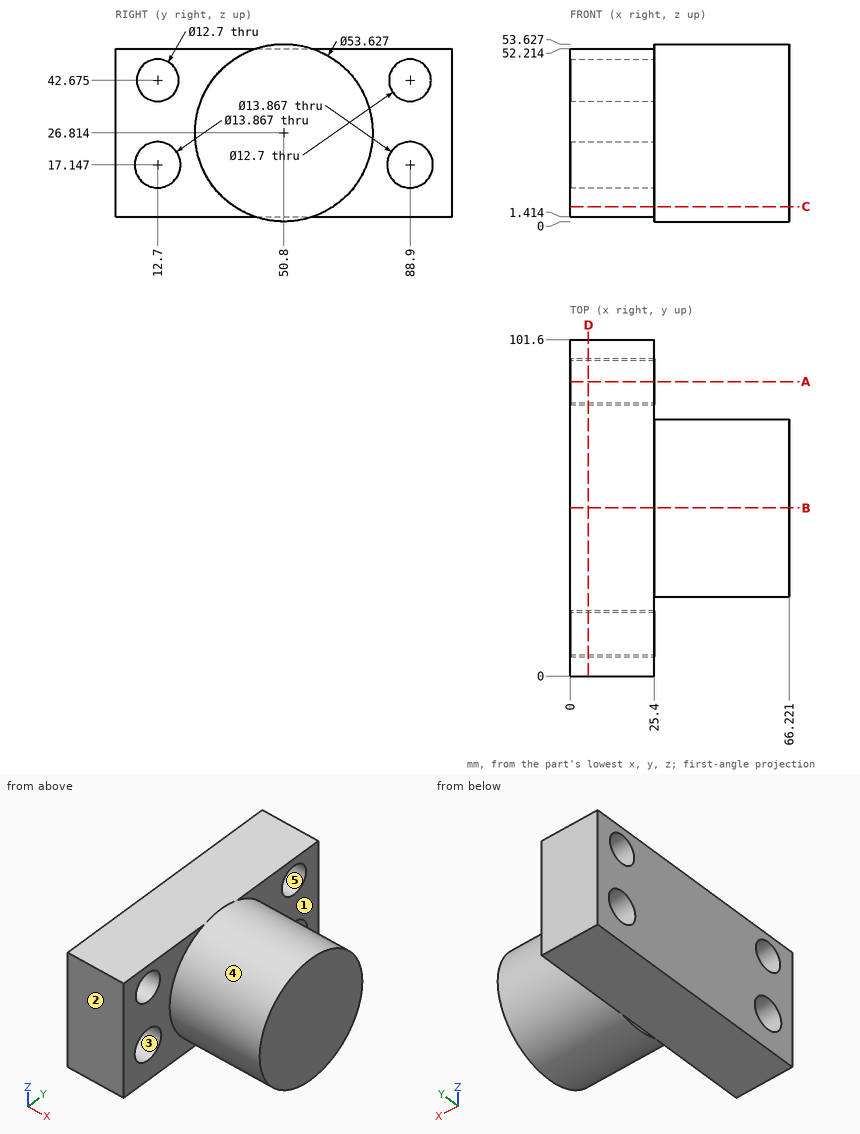
The figure shows three views and two pictorial views of one solid part (mm, origin at its lowest corner). Answer the questions. A direction names the side the tool comes from. Coordinates: 2 decimals unless noted, no trailing zeros. Loops run counter-clockwise (first coordinate to the right, second up) from the corner with the lowest first, then second, coordinate; pieces in that order, holes last. Notation, with made-up numbers: (-30.5, 62) - (-22.5, 62) arc R13 cw to (-22.5, 82) - close; hole circle Ø2 at (8.25, 81). An arc over 180 degrees is marked (long way). Write item = value, one per line.
1) Find the intervals of material crossed by line 1 along Z through (x, y) = (9, 12.7) (1 decimal); line 2 along Y through (x, z) = (6, 43); line 3 along Z through (x, y) = (15, 12) (1 decimal), in increasing order.
Responses:
line_1 = 1.4 to 10.2, 24.1 to 36.3, 49 to 52.2
line_2 = 0 to 6.36, 19.04 to 82.56, 95.24 to 101.6
line_3 = 1.4 to 10.2, 24 to 36.4, 49 to 52.2
2) Section A-A (y = 88.9) is taken. Determine the outline of the cut face in (x, z) (1 decimal).
Responses:
outline = (0, 1.4) - (25.4, 1.4) - (25.4, 10.2) - (0, 10.2) - close; (0, 24.1) - (25.4, 24.1) - (25.4, 36.3) - (0, 36.3) - close; (0, 49) - (25.4, 49) - (25.4, 52.2) - (0, 52.2) - close
3) Section C-C (z = 4.5) is taken. Determine the outline of the cut face in (x, y), plus the area to 3 significant figures.
Responses:
outline = (0, 0) - (25.4, 0) - (25.4, 35.93) - (66.22, 35.93) - (66.22, 65.67) - (25.4, 65.67) - (25.4, 101.6) - (0, 101.6) - close
area = 3,790 mm^2
4) Each of these flat-tipped pins is pushed along its axis until it touches: P1, Ø3, axis at x = 57, y = 27.5, coming from the +Z side (1 decimal); P2, Ø22, axis at y = 88.9, z = 17.15, coming from the +X side; P3, Ø12.5, axis at x = 14, y = 58, coming from the -Z side; P4, Ø11.5, axis at y = 12.7, z = 42.67, coming from the -X side. Where does it stop, or does it pass through?
Responses:
P1 = 42.4
P2 = 25.4
P3 = 1.41
P4 = through
5) Section D-D (x = 5.5) is taken. Count the separate pieces of the cut face and the enclosed holes in it, plus the area to 3 significant figures.
Responses:
separate_pieces = 1
enclosed_holes = 4
area = 4,610 mm^2
6) Determine the mould class of the marked faces 1, 2 and 3 for opening direction Y: pulls with the +Y half, pulls with the -Y half, needs draft (parallel to the pull), parting line crosses it, or undercut.
Responses:
face_1 = needs draft
face_2 = pulls with the -Y half
face_3 = undercut
7) Section B-B (y = 50.8) is taken. Determine the outline of the cut face in (x, z), plus the area to 3 significant figures.
Responses:
outline = (0, 1.41) - (25.4, 1.41) - (25.4, 0) - (66.22, 0) - (66.22, 53.63) - (25.4, 53.63) - (25.4, 52.21) - (0, 52.21) - close
area = 3,480 mm^2
8) Which of the six approach directions +Z, -Z, +X, -X, +Y, -Y give full straight-line access (tool end or side, diameter ignored) to the marked faces 4 and 5?
Responses:
face_4 = +X
face_5 = +X, -X
